```python
from build123d import *

# Parameters (mm, degrees)
BOSS_EXTRUDE1_DEPTH = 125
FILLET1_R           = 1.5
FILLET2_R           = 1.5
SKETCH2_R           = 2.75
CUT_EXTRUDE1_DEPTH  = 2.5


with BuildPart() as part:
    # Sketch1 → Boss-Extrude1 (new body)
    with BuildSketch(Plane(origin=(0, 0, 0), x_dir=(1, 0, 0), z_dir=(0, 1, 0))):
        Polygon((0, 0), (0, 35), (1.5, 35), (1.5, 1.5), (18, 1.5), (18, 0), align=None)
    extrude(amount=BOSS_EXTRUDE1_DEPTH)

    # Fillet1
    fillet1_edges = [part.edges().sort_by_distance(p)[0] for p in [
        (1.5, 62.5, -1.5),
    ]]
    fillet(fillet1_edges, radius=FILLET1_R)

    # Fillet2
    fillet2_edges = [part.edges().sort_by_distance(p)[0] for p in [
        (0, 62.5, 0),
    ]]
    fillet(fillet2_edges, radius=FILLET2_R)

    # Sketch2 → Cut-Extrude1 (cut, through all)
    with BuildSketch(Plane(origin=(1.5, 0, 0), x_dir=(0, 0, -1), z_dir=(1, 0, 0))):
        with Locations((30, 110)):
            Circle(SKETCH2_R)
        with Locations((30, 15)):
            Circle(SKETCH2_R)
    extrude(amount=-CUT_EXTRUDE1_DEPTH, mode=Mode.SUBTRACT)


solid = part.part
```
Part model, mm, in its own coordinate system. A direction names the side the tool comes from. Coordinates: 2 decimals unless noted, no trailing zeros. Loops run counter-clockwise (first coordinate to the right, second up) from the corner with the lowest first, then second, coordinate; pieces in that order, holes last. Notation, with made-up numbers: (31.25, 34) - (52.25, 34) arc R15 cw to (52.25, 39) - close; hole circle Ø9 at (-32.5, 75). An arc over 180 degrees is marked (long way). Write item = value, one per line. Start each with the question number.
Item 1: Flat gauge pins, fed straight in: pin 1 Ø3 at (x, y) = (11, 78.5) entering from -Z; pin 2 Ø16 at (y, z) = (63, -20.5) entering from +X; pin 3 Ø4 at (x, z) = (4, -12) entering from -Y; pin 4 Ø1.5 at (x, y) = (2.5, 82.5) entering from -Z. Where does each tip first touch, or does it go through?
Item 2: Cut at B-B, the plane z = -30. Give the cut face in (x, y), and give its area (3 significant figures).
Item 3: 3-axis set-ups, long thin cutter, end or side, ignore diameter. For faces 1 (the cylindrical face through (0.76, 15.121, -27.253)), 2 (the flat face through (10, 62, -1.5)): which of +Z, -Z, +X, -X, +Y, -Y reach the whole face in a straight line?
Item 4: Wall check: L1, parallel to Y at x = 0.7, z = -30; L2, parallel to X at y = 67, z = -30.5; L3, parallel to Z at x = 15.25, y = 66.5. Give the ranges that are in metal, low to high. Write a range as from..to.
Item 5: Cut at C-C, the plane y = 85. Give the cut face in (x, z), and give its area (4 significant figures).
Item 6: Cut at D-D, the plane x = 4.5. Give the cut face in (y, z).
Item 7: Mould opens along Y. For faces 3 (the flat face through (0, 62, -18)), 4 (the flat face through (1, 125, -12)), 5 (the cylindrical face through (0.76, 107.315, -29.404)) say: released by +Y, released by -Y, zero draft, split by the parting line, or undercut.
Item 8: Cut at A-A, the plane y = 15. Give the cut face in (x, z), and give its area (3 significant figures).
The answers:
q1.pin_1 = -1.5
q1.pin_2 = 1.5
q1.pin_3 = through
q1.pin_4 = -2.17
q2.outline = (0, 0) - (1.5, 0) - (1.5, 12.25) - (0, 12.25) - close; (0, 17.75) - (1.5, 17.75) - (1.5, 107.25) - (0, 107.25) - close; (0, 112.75) - (1.5, 112.75) - (1.5, 125) - (0, 125) - close
q2.area = 171 mm2
q3.face_1 = +X, -X
q3.face_2 = -Z, +X, +Y, -Y
q4.L1 = 0..12.25, 17.75..107.25, 112.75..125
q4.L2 = 0..1.5
q4.L3 = -1.5..0
q5.outline = (0, -35) - (1.5, -35) - (1.5, -3) arc R1.5 cw to (3, -1.5) - (18, -1.5) - (18, 0) - (1.5, 0) arc R1.5 ccw to (0, -1.5) - close
q5.area = 77.25 mm2
q6.outline = (0, -1.5) - (125, -1.5) - (125, 0) - (0, 0) - close
q7.face_3 = zero draft
q7.face_4 = released by +Y
q7.face_5 = undercut
q8.outline = (0, -35) - (1.5, -35) - (1.5, -32.75) - (0, -32.75) - close; (0, -27.25) - (1.5, -27.25) - (1.5, -3) arc R1.5 cw to (3, -1.5) - (18, -1.5) - (18, 0) - (1.5, 0) arc R1.5 ccw to (0, -1.5) - close
q8.area = 69.0 mm2
